from build123d import *

# Parameters (mm, degrees)
SKETCH1_W           = 10
SKETCH1_H           = 1.8
SKETCH1_W_2         = 1.9
SKETCH1_H_2         = 4.7
BOSS_EXTRUDE1_DEPTH = 180
SKETCH2_W           = 22
SKETCH2_H           = 1.8
BOSS_EXTRUDE2_DEPTH = 20
CHAMFER1_SIZE       = 7
CHAMFER1_SIZE2      = 4.7


with BuildPart() as part:
    # Sketch1 → Boss-Extrude1 (new body)
    with BuildSketch(Plane.XY):
        with Locations((5, 0.9)):
            Rectangle(SKETCH1_W, SKETCH1_H)
        with Locations((5, 4.15)):
            Rectangle(SKETCH1_W_2, SKETCH1_H_2)
    extrude(amount=BOSS_EXTRUDE1_DEPTH)

    # Sketch2 → Boss-Extrude2 (add)
    with BuildSketch(Plane.XY.offset(180)):
        with Locations((5, 0.9)):
            Rectangle(SKETCH2_W, SKETCH2_H)
    extrude(amount=-BOSS_EXTRUDE2_DEPTH)

    # Chamfer1
    chamfer1_edges = [part.edges().sort_by_distance(p)[0] for p in [
        (5, 6.5, 180),
    ]]
    chamfer1_side = [part.faces().sort_by_distance(p)[0] for p in [
        (5, 6.5, 90),
    ]]
    chamfer(chamfer1_edges, length=CHAMFER1_SIZE, length2=CHAMFER1_SIZE2, reference=chamfer1_side[0])


solid = part.part
Here's how the part is built. I have some questions about the finished solid (model axes, mm). A direction names the side the tool comes from. Round coordinates to 2 decimals unless told otherwise and drop trailing zeros. Write each loop counter-clockwise with the first axis right and the second up, starting at its lowest first coordinate (ties: lowest second). Pieces come first, ordered by that corner, then holes.
1. I need wall thicknesses on L1, parallel to Y at x = 7.5, z = 32; L2, parallel to X at y = 3.25, z = 12. Which ranges of each line are inside material? Lowest first, please.
2. Suppose I cut it at B-B (x = 14.25). List the corners of the cut face in (y, z) for me, and give its area (3 significant figures).
3. Suppose I cut it at A-A (z = 57). List the corners of the cut face in (x, y) for me.
4. For faces 1 (the flat face through (4.05, 4, 89)), 2 (the flat face through (5.95, 4, 89)), 3 (the flat face through (4.987, 4.117, 176.549)), which set-ups out of +Z, -Z, +X, -X, +Y, -Y let a thin tool reach every point of the face, with its end or its side?
5. Will these pins go through, and if not, where does the flat tip stop? pin 1 Ø3 at (x, z) = (0, 108.5) entering from +Y; pin 2 Ø0.5 at (x, y) = (12, 1) entering from -Z; pin 3 Ø3 at (y, z) = (2, 46.5) entering from -X.
6. Suppose I cut it at C-C (y = 5). List the corners of the cut face in (x, z) for me, and give its area (3 significant figures).
Answer sheet:
1. L1: y = 0 to 1.8
1. L2: x = 4.05 to 5.95
2. outline: (0, 160) - (1.8, 160) - (1.8, 180) - (0, 180) - close
2. area: 36.0 mm2
3. outline: (0, 0) - (10, 0) - (10, 1.8) - (5.95, 1.8) - (5.95, 6.5) - (4.05, 6.5) - (4.05, 1.8) - (0, 1.8) - close
4. face 1: +Z, -Z, -X, +Y
4. face 2: +Z, -Z, +X, +Y
4. face 3: +Z, +X, -X, +Y
5. pin 1: stops at y = 1.8
5. pin 2: stops at z = 160
5. pin 3: stops at x = 0
6. outline: (4.05, 0) - (5.95, 0) - (5.95, 175.23) - (4.05, 175.23) - close
6. area: 333 mm2
